Design review of the part built by this model. Coordinates are the model's own, in mm. Face numbers are marked on the shaded views. A direction names the side the tool comes from. Coordinates: 2 decimals unless noted, no trailing zeros. Write each loop counter-clockwise with the first axis right and the second up, starting at its lowest first coordinate (ties: lowest second). Pieces come first, ordered by that corner, then holes. Notation, with made-up numbers: (15, -27.75) -> (38, -27.75) arc R18 cw to (38, -22.75) -> close; hole circle Ø8 at (75.5, 36). An arc over 180 degrees is marked (long way). One line per question, with ' | ' between items. Start each with the question number.
Q1. Wall thickness on probe 1 along X at (y, z) = (-5.85, 9.6); probe 2 along Y at (x, z) = (0, 9.75); probe 3 along Z at (x, y) = (19, -4.25): over which ranges is each line inside the solid? List them lowest first.
Q2. Add section B-B on z = 6.75. State the section outline as (x, y) points.
Q3. For the marked faces 4, 5, 6 and 7, list the 3-axis set-ups (+Z, -Z, +X, -X, +Y, -Y) from which the entire face can be reached by the end or side of a thin tool; tool diameter is ignored.
Q4. For P1, Ø2.5, axis at x = 77.5, z = 11.5, coming from the +Y side; P2, Ø4, axis at x = 57, z = 12.5, coming from the +Y side; P3, Ø1, axis at y = 0.5, z = 3, coming from the +X side, all flat-tipped, find the tip position at first contact; note any pin that passes through.
Q5. Draft analysis for pull direction X (two halves, no side actions). For the marked faces 1, 2 and 3, state which applies: pulls with the +X half, pulls with the -X half, needs draft (parallel to the pull), parting line crosses it, or undercut.
Q6. Add section A-A on x = 0. State the section outline as (y, z) points.
from build123d import *

# Parameters (mm, degrees)
ESQUISSE1_R                  = 5.95
ESQUISSE1_R_2                = 4.45
EXTRU_MINCE1_DEPTH           = 19.2
EXTRU_MINCE1_2_DEPTH         = 19.2
EXTRU_MINCE1_3_DEPTH         = 19.2
ESQUISSE3_W                  = 20
ESQUISSE3_H                  = 19.2
ESQUISSE3_W_2                = 40
BOSS_EXTRU_1_DEPTH           = 1.1
CONG_1_R                     = 10
ENL_V_MAT_EXTRU_1_DEPTH      = 83.99724393
ENL_V_MAT_EXTRU_1_DEPTH_BACK = 83.99724393
ESQUISSE4_W                  = 5
ESQUISSE4_H                  = 3
ESQUISSE5_R                  = 1.5
ENL_V_MAT_EXTRU_4_DEPTH      = 83.99724393


with BuildPart() as part:
    # Esquisse1 → Extru.-Mince1 (new body)
    with BuildSketch(Plane.XY):
        Circle(ESQUISSE1_R)
        Circle(ESQUISSE1_R_2, mode=Mode.SUBTRACT)
    extrude(amount=EXTRU_MINCE1_DEPTH)



with BuildPart() as body_2:
    # Esquisse1 → Extru.-Mince1 2 (new body)
    with BuildSketch(Plane.XY):
        with Locations((30, 0)):
            Circle(ESQUISSE1_R)
        with Locations((30, 0)):
            Circle(ESQUISSE1_R_2, mode=Mode.SUBTRACT)
    extrude(amount=EXTRU_MINCE1_2_DEPTH)


with BuildPart() as body_3:
    # Esquisse1 → Extru.-Mince1 3 (new body)
    with BuildSketch(Plane.XY):
        with Locations((60, 0)):
            Circle(ESQUISSE1_R)
        with Locations((60, 0)):
            Circle(ESQUISSE1_R_2, mode=Mode.SUBTRACT)
    extrude(amount=EXTRU_MINCE1_3_DEPTH)


with BuildPart() as part_1:
    add(part.part)

    add(body_2.part)  # Boss.-Extru.1 merges body 2

    add(body_3.part)  # Boss.-Extru.1 merges body 3
    # Esquisse3 → Boss.-Extru.1 (add)
    with BuildSketch(Plane(origin=(0, -5, 0), x_dir=(1, 0, 0), z_dir=(0, 1, 0))):
        with Locations((-10, -9.6)):
            Rectangle(ESQUISSE3_W, ESQUISSE3_H)
        with Locations((10, -9.6)):
            Rectangle(ESQUISSE3_W, ESQUISSE3_H)
        with Locations((30, -9.6)):
            Rectangle(ESQUISSE3_W, ESQUISSE3_H)
        with Locations((60, -9.6)):
            Rectangle(ESQUISSE3_W_2, ESQUISSE3_H)
    extrude(amount=-BOSS_EXTRU_1_DEPTH)

    # Congé1
    # the kernel refuses this fillet: 10 mm, written as the material it adds along each edge
    with BuildSketch(Plane(origin=(-3.225290685, -5, 19.2), x_dir=(-0.33303824301553114, 0.9429133198174305, 0), z_dir=(0, 0, -1)), Plane(origin=(26.774709315, -5, 19.2), x_dir=(-0.33303824301553103, 0.9429133198174305, 0), z_dir=(0, 0, -1)), Plane(origin=(56.774709315, -5, 19.2), x_dir=(-0.3330382430155325, 0.9429133198174301, 0), z_dir=(0, 0, -1))) as cong_1_piece_1:
        with BuildLine():
            CenterArc((13.399198301, -7.90985002), CONG_1_R, 127.722343038, 71.730945551)
            Line((3.970065103, -11.24023245), (0, 0))
            ThreePointArc((0, 0), (3.640421456, -1.243639238), (7.280842913, 0))
        make_face()
    extrude(amount=19.2)
    with BuildSketch(Plane(origin=(3.225290685, -5, 19.2), x_dir=(0.33303824301553153, 0.9429133198174304, 0), z_dir=(0, 0, -1))) as cong_1_piece_2:
        with BuildLine():
            CenterArc((13.399198301, 7.90985002), CONG_1_R, 160.546711411, 71.730945551)
            Line((3.970065103, 11.24023245), (0, 0))
            ThreePointArc((0, 0), (3.640421456, 1.243639238), (7.280842913, 0))
        make_face()
    extrude(amount=19.2)
    with BuildSketch(Plane(origin=(33.225290685, -5, 19.2), x_dir=(1, 0, 0), z_dir=(0, 0, -1)), Plane(origin=(63.225290685, -5, 19.2), x_dir=(1, 0, 0), z_dir=(0, 0, -1))) as cong_1_piece_3:
        with BuildLine():
            CenterArc((11.920748402, -10), CONG_1_R, 90, 71.730945551)
            ThreePointArc((2.424799131, -6.865203762), (2.385043568, -3.018422454), (0, 0))
            Line((0, 0), (11.920748402, 0))
        make_face()
    extrude(amount=19.2)

    # Esquisse4 → Enlèv. mat.-Extru.1 (cut, two sides: drawn at the far end of the back side and taken through both)
    with BuildSketch(Plane(origin=(0, -5, 0), x_dir=(1, 0, 0), z_dir=(0, 1, 0)).offset(-ENL_V_MAT_EXTRU_1_DEPTH_BACK)):
        with Locations((-11, -15.2)):
            Rectangle(ESQUISSE4_W, ESQUISSE4_H)
        with Locations((11, -15.2)):
            Rectangle(ESQUISSE4_W, ESQUISSE4_H)
        with Locations((19, -15.2)):
            Rectangle(ESQUISSE4_W, ESQUISSE4_H)
        with Locations((41, -15.2)):
            Rectangle(ESQUISSE4_W, ESQUISSE4_H)
        with Locations((49, -15.2)):
            Rectangle(ESQUISSE4_W, ESQUISSE4_H)
        with Locations((71, -15.2)):
            Rectangle(ESQUISSE4_W, ESQUISSE4_H)
    extrude(amount=ENL_V_MAT_EXTRU_1_DEPTH + ENL_V_MAT_EXTRU_1_DEPTH_BACK, mode=Mode.SUBTRACT)

    # Esquisse5 → Enlèv. mat.-Extru.4 (cut, through all)
    with BuildSketch(Plane(origin=(0, -5, 0), x_dir=(1, 0, 0), z_dir=(0, 1, 0))):
        with BuildLine():
            ThreePointArc((79.073019543, -9.6), (78.494574401, -8.416472796), (77.205370686, -8.145753007))
            Line((77.205370686, -8.145753007), (77.940668401, -11.054246993))
            ThreePointArc((77.940668401, -11.054246993), (78.756546747, -10.521554858), (79.073019543, -9.6))
        make_face()
        with BuildLine():
            Line((77.940668401, -11.054246993), (77.205370686, -8.145753007))
            ThreePointArc((77.205370686, -8.145753007), (76.11877255, -9.967648858), (77.940668401, -11.054246993))
        make_face()
        with Locations(Location((-17.573019543, -9.6, 0), (0, 0, 270))):
            Circle(ESQUISSE5_R)
    extrude(amount=-ENL_V_MAT_EXTRU_4_DEPTH, mode=Mode.SUBTRACT)


solid = part_1.part
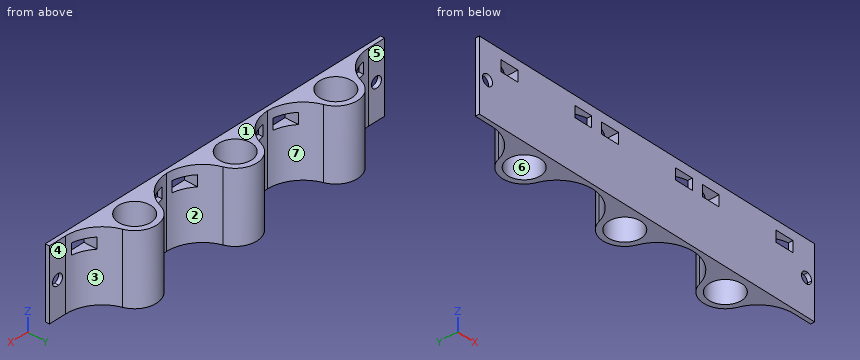
Output values:
1) probe 1: x = -20 to -19.07, -16.07 to 76.07, 79.07 to 80 | probe 2: y = -6.1 to -4.45, 4.45 to 5.95 | probe 3: z = 0 to 13.7, 16.7 to 19.2
2) outline: (-20, -6.1) -> (80, -6.1) -> (80, -5) -> (75.15, -5) arc R10 cw to (65.65, 1.87) arc R5.95 ccw to (54.35, 1.87) arc R10 cw to (45, -5) arc R10 cw to (35.65, 1.87) arc R5.95 ccw to (24.35, 1.87) arc R10 cw to (15, -5) arc R10 cw to (5.65, 1.87) arc R5.95 ccw to (-5.65, 1.87) arc R10 cw to (-15.15, -5) -> (-20, -5) -> close; hole circle Ø8.9 at (0, 0); hole circle Ø8.9 at (30, 0); hole circle Ø8.9 at (60, 0)
3) face 4: +Z, -Z, +X, +Y | face 5: +Z, -Z, -X, +Y | face 6: +Z, -Z | face 7: +Z, -Z, +Y
4) P1: stops at y = -5 | P2: stops at y = 5.87 | P3: stops at x = 66.49
5) face 1: needs draft | face 2: undercut | face 3: pulls with the +X half
6) outline: (-6.1, 0) -> (-4.45, 0) -> (-4.45, 19.2) -> (-6.1, 19.2) -> close; (4.45, 0) -> (5.95, 0) -> (5.95, 19.2) -> (4.45, 19.2) -> close
